```python
from build123d import *

# Parameters (mm, degrees)
F1_DEPTH = 3


with BuildPart() as f1:
    # F0 (on Front) → F1 (new body)
    with BuildSketch(Plane.XZ):
        with BuildLine():
            Line((5, 20), (-5, 20))
            ThreePointArc((-5, 20), (-12.0710678119, 17.0710678119), (-15, 10))
            Line((-15, 10), (-15, -10))
            ThreePointArc((-15, -10), (-12.0710678119, -17.0710678119), (-5, -20))
            Line((-5, -20), (5, -20))
            ThreePointArc((5, -20), (12.0710678119, -17.0710678119), (15, -10))
            Line((15, -10), (15, 10))
            ThreePointArc((15, 10), (12.0710678119, 17.0710678119), (5, 20))
        make_face()
    extrude(amount=F1_DEPTH)

    # F4 (on offset) → F5 (revolve)
    with BuildSketch(Plane.YZ):
        with BuildLine():
            Line((-33, -10), (-3, -10))
            Line((-3, -10), (-3, -6))
            Line((-3, -6), (-3, -2.8667848092))
            Line((-3, -2.8667848092), (-6.0189967044, -6))
            Line((-6.0189967044, -6), (-23.9476568219, -6))
            ThreePointArc((-23.9476568219, -6), (-24.9406776462, -5.8308849575), (-25.8217419646, -5.3426064283))
            Line((-25.8217419646, -5.3426064283), (-29.1782580354, -2.6573935717))
            ThreePointArc((-29.1782580354, -2.6573935717), (-30.0593223538, -2.1691150425), (-31.0523431781, -2))
            Line((-31.0523431781, -2), (-32, -2))
            ThreePointArc((-32, -2), (-32.7071067812, -2.2928932188), (-33, -3))
            Line((-33, -3), (-33, -10))
        make_face()
    revolve(axis=Axis((0, -24.5992667091, -10), (0, -1, 0)))


solid = f1.part
```
Input: part model. Units: mm. Frame: model coordinates. A direction names the side the tool comes from. Round coordinates to 2 decimals unless told otherwise and drop trailing zeros. Loops run counter-clockwise (first coordinate to the right, second up) from the corner with the lowest first, then second, coordinate; pieces in that order, holes last.
1) Section query B-B on y = -16.5. Return the cut outline in (x, z).
Ans:
outline: circle Ø8 at (0, -10)
2) Section query A-A on x = 0. Return the cut outline in (y, z), plus the area to 3 significant figures.
Ans:
outline: (-33, -17) arc R1 ccw to (-32, -18) - (-31.05, -18) arc R3 ccw to (-29.18, -17.34) - (-25.82, -14.66) arc R3 cw to (-23.95, -14) - (-6.02, -14) - (-3, -17.13) - (-3, -20) - (0, -20) - (0, 20) - (-3, 20) - (-3, -2.87) - (-6.02, -6) - (-23.95, -6) arc R3 cw to (-25.82, -5.34) - (-29.18, -2.66) arc R3 ccw to (-31.05, -2) - (-32, -2) arc R1 ccw to (-33, -3) - close
area: 413 mm2
3) Material intervals for line 1 (Z direction, x = -1.25, y = -25); line 2 (Y direction, x = -7, z = -14.5); line 3 (Y direction, x = -0.75, z = -16.5), sorted ascending.
Ans:
line 1: z = -14 to -6
line 2: y = -3 to 0
line 3: y = -33 to -28.18, -3.57 to 0
4) Section query C-C on z = 17. Return the cut outline in (x, y).
Ans:
outline: (-12.14, -3) - (12.14, -3) - (12.14, 0) - (-12.14, 0) - close
5) Pull-direction query (Y, two-part tool) for faces 1 (the flat face through (0, -33, -10)), 2 (the flat face through (-15, -1, 0)), 3 (the cylindrical face through (2.4, -15.1, -13.2)); classes: released by +Y, released by -Y, zero draft, split by the parting line, or undercut.
Ans:
face 1: released by -Y
face 2: zero draft
face 3: undercut
6) Set-up query: faces 4 (the flat face through (0, 0, 0)), 5 (the cylindrical face through (7.81, -31.53, -11.73)), 6 (the conical face through (-1.25, -5.87, -6.04)). Return all of +Z, -Z, +X, -X, +Y, -Y with unobstructed straight access to the full face (end or side cutting, diameter ignored); none if empty.
Ans:
face 4: +Z, -Z, +X, -X, +Y
face 5: -Y
face 6: none
7) Section query D-D on z = 10.5. Return the cut outline in (x, y), plus the area to 3 significant figures.
Ans:
outline: (-14.99, -3) - (14.99, -3) - (14.99, 0) - (-14.99, 0) - close
area: 89.9 mm2
8) Pin query (flat end, axial travel): pin 1 (15 mm diameter, centred on x = -1.5, z = 9.5, fed in from -Y); pin 2 (1 mm diameter, centred on x = -6.5, y = -26.5, fed in from +Z); pin 3 (5 mm diameter, centred on y = -25, z = -4.5, fed in from +X); pin 4 (10 mm diameter, centred on y = -21.5, z = -5, fed in from +X). Return the tip coordinate at first contact, or that it passes through.
Ans:
pin 1: stops at y = -3
pin 2: passes through
pin 3: stops at x = 3.93
pin 4: stops at x = 4
